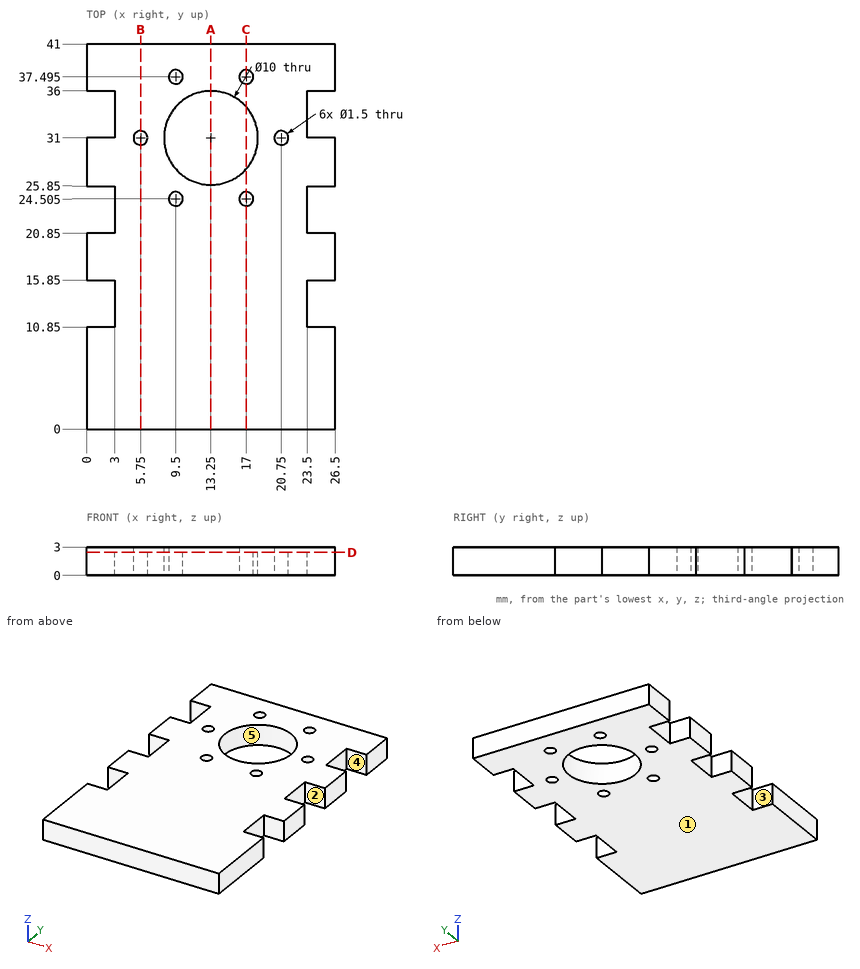
Here's the drawing with two shaded views (mm, measured from the low corner). I have some questions. A direction names the side the tool comes from. Round coordinates to 2 decimals unless told otherwise and drop trailing zeros. Loops run counter-clockwise (first coordinate to the right, second up) from the corner with the lowest first, then second, coordinate; pieces in that order, holes last. Notation, with made-up numbers: M -28,-1 L 14,-1 A12 ccw 14,22 Z; hole C 4,-24.5 d9. An arc over 180 degrees is marked long. Answer as a JSON object with one key per item and string values. Group by question number.
Q1. On a 3-axis mill with a long thin cutter (end or side, diameter ignored), from which of +Z, -Z, +X, -X, +Y, -Y can I reach the whole of each face in a straight line? I mean the marked faces 1, 2 and 3. Say none if no direction works.
Q2. We'd pull the mould along X, two halves only. Please class the marked faces 4 and 5: +X half, -X half, draft (parallel to the pull), parting line (faces both ways), or undercut.
Q3. Please list where these lines run through material, in increasing order: L1, parallel to Y at x = 2.5, z = 1.4; L2, parallel to Y at x = 5.75, z = 2.4; L3, parallel to X at y = 30.5, z = 1.9 (1 decimal).
Q4. Imagine slicing it at B-B, the plane x = 5.75. Please give me the cut outline in (y, z), then the cut area to 4 significant figures.
Q5. Imagine slicing it at D-D, the plane z = 2.45. Count the separate pieces of the cut face and the enclosed holes in it, then the cut area to 3 significant figures.
Q6. Imagine slicing it at C-C, the plane x = 17. Please give me the cut outline in (y, z) (1 decimal).
Q7. Will these pins go through, and if not, where does the flat tip stop? pin 1 (13 mm diameter, centred on x = 13.25, y = 31, fed in from -Z); pin 2 (1.5 mm diameter, centred on y = 34.5, z = 1.5, fed in from +X).
Q8. Imagine slicing it at A-A, the plane x = 13.25. Please give me the cut outline in (y, z).
Findings:
{
 "1": {"face 1": "-Z, +X, -X, +Y, -Y", "face 2": "+Z, -Z, +X", "face 3": "+Z, -Z, -X"},
 "2": {"face 4": "draft", "face 5": "undercut"},
 "3": {"L1": "y = 0 to 10.85, 15.85 to 20.85, 25.85 to 31, 36 to 41", "L2": "y = 0 to 30.25, 31.75 to 41", "L3": "x = 0 to 5.2, 6.3 to 8.3, 18.2 to 20.2, 21.3 to 26.5"},
 "4": {"outline": "M 0,0 L 30.25,0 L 30.25,3 L 0,3 Z; M 31.75,0 L 41,0 L 41,3 L 31.75,3 Z", "area": "118.5 mm2"},
 "5": {"separate pieces": "1", "enclosed holes": "7", "area": "907 mm2"},
 "6": {"outline": "M 0,0 L 23.8,0 L 23.8,3 L 0,3 Z; M 25.3,0 L 27.7,0 L 27.7,3 L 25.3,3 Z; M 34.3,0 L 36.7,0 L 36.7,3 L 34.3,3 Z; M 38.2,0 L 41,0 L 41,3 L 38.2,3 Z"},
 "7": {"pin 1": "stops at z = 0", "pin 2": "stops at x = 23.5"},
 "8": {"outline": "M 0,0 L 26,0 L 26,3 L 0,3 Z; M 36,0 L 41,0 L 41,3 L 36,3 Z"}
}
